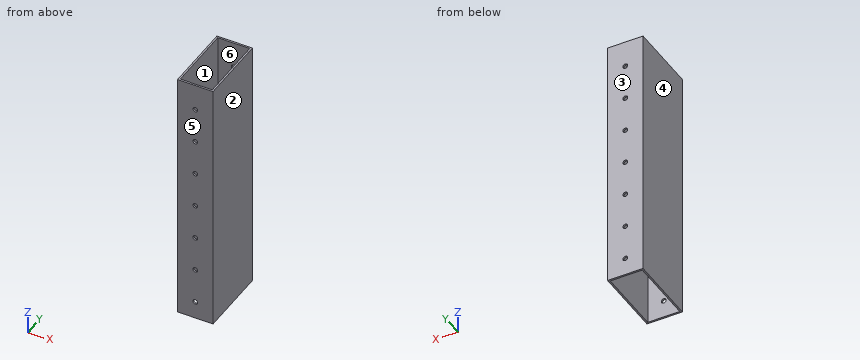
Autodesk Inventor part; units mm, degrees
ref_plane "YZ Plane" through (0, 0, 0) normal (1, 0, 0) x (0, 1, 0)
ref_plane "XZ Plane" through (0, 0, 0) normal (0, 1, 0) x (-1, 0, 0)
ref_plane "XY Plane" through (0, 0, 0) normal (0, 0, 1) x (1, 0, 0)
sketch "Sketch1" plane through (0, 0, 0) normal (0, 0, 1) x (1, 0, 0)
  line L0 (-12.1708, 16.0073) -> (13.2292, 16.0073)
  line L1 (13.2292, 16.0073) -> (13.2292, -34.7927)
  line L2 (13.2292, -34.7927) -> (-12.1708, -34.7927)
  line L3 (-12.1708, -34.7927) -> (-12.1708, 16.0073)
  line L4 (11.9592, 14.7373) -> (-10.9008, 14.7373)
  line L5 (-10.9008, 14.7373) -> (-10.9008, -33.5227)
  line L6 (-10.9008, -33.5227) -> (11.9592, -33.5227)
  line L7 (11.9592, -33.5227) -> (11.9592, 14.7373)
  point P0 (0, 0)
  dimension "d0" = 25.4
  dimension "d1" = 50.8
  dimension "d2" = 1.27
extrude "Extrusion1" add sketch "Sketch1" along normal blind 184.15
sketch "Sketch2" plane through (-12.1708, 16.0073, 0) normal (0, 1, 0) x (1, 0, 0)
  circle A0 centre (12.7, -12.7) radius 1.7272
  line L0 (25.4, 0) -> (0, 0)
  line L1 (0, 0) -> (0, -184.15)
  point P0 (12.1708, 0)
  dimension "d5" = 3.4544
  dimension "d6" = 12.7
  dimension "d7" = 12.7
extrude "Extrusion2" cut sketch "Sketch2" against normal through all
pattern_linear "Rectangular Pattern1" count 71 spacing 25.4 along (0, 0, 1) of "Extrusion2"
equation "\"d10\" = d14"
equation "\"d13\" = 711.2"
equation "\"d14\" = d13"
properties part number "VersaFrame_IndexSupp"
Geometry: final body of the model. Coordinates: model frame, mm. Face numbers are marked on the shaded views. A direction names the side the tool comes from. Coordinates: 2 decimals unless noted, no trailing zeros. Order: outer loops, then holes, each group sorted by start corner. A loop starts at its lowest first (then second) coordinate and runs counter-clockwise, first axis right, second up. Notation, with made-up numbers: M -29.5,29 L 7.5,29 A22 ccw 7.5,53 Z; hole C 76,46 d11. An arc over 180 degrees is marked long. Answer in a Markdown table with one row per item. Add a question column.
Q1. Line query: L1, parallel to X at y = -34.5, z = 165.1; L2, parallel to X at y = 15, z = 114; L3, parallel to Y at x = 9.25, z = 120. Output: solid intervals per line, ascending.
Q2. Contact query for a flat-ended pin moving along its axis: P1, Ø3, axis at x = 0.53, z = 12.7, coming from the +Y side. Output: stop coordinate, or through.
Q3. Mould query, pull axis Y, two halves, no side actions, for the marked faces 3, 4, 5 and 6. Classes: released by +Y, released by -Y, zero draft, split by the parting line, or undercut.
Q4. Section query C-C on x = 8.75. Return the cut outline in (y, z).
Q5. Section query B-B on y = 11.5. Return the cut outline in (x, z), and give its area (3 significant figures).
Q6. Section query A-A on z = 12.7. Return the cut outline in (x, y).
Q7. Section query D-D on z = 48.5. Return the cut outline in (x, y).
Q8. Reachability of the marked faces 1 and 2 from +Z, -Z, +X, -X, +Y, -Y: full face, straight path, thin tool, end or side. Return the list, or none.
Completed:
| question | item | result |
|---|---|---|
| 1 | L1 | x = -12.17 to -1.2, 2.26 to 13.23 |
| 1 | L2 | x = -12.17 to -1.17, 2.23 to 13.23 |
| 1 | L3 | y = -34.79 to -33.52, 14.74 to 16.01 |
| 2 | P1 | passes through |
| 3 | face 3 | released by +Y |
| 3 | face 4 | zero draft |
| 3 | face 5 | released by -Y |
| 3 | face 6 | undercut |
| 4 | outline | M -34.79,0 L -33.52,0 L -33.52,184.15 L -34.79,184.15 Z; M 14.74,0 L 16.01,0 L 16.01,184.15 L 14.74,184.15 Z |
| 5 | outline | M -12.17,0 L -10.9,0 L -10.9,184.15 L -12.17,184.15 Z; M 11.96,0 L 13.23,0 L 13.23,184.15 L 11.96,184.15 Z |
| 5 | area | 468 mm2 |
| 6 | outline | M -12.17,-34.79 L -1.2,-34.79 L -1.2,-33.52 L -10.9,-33.52 L -10.9,14.74 L -1.2,14.74 L -1.2,16.01 L -12.17,16.01 Z; M 2.26,-34.79 L 13.23,-34.79 L 13.23,16.01 L 2.26,16.01 L 2.26,14.74 L 11.96,14.74 L 11.96,-33.52 L 2.26,-33.52 Z |
| 7 | outline | M -12.17,-34.79 L 13.23,-34.79 L 13.23,16.01 L -12.17,16.01 Z; hole M -10.9,-33.52 L 11.96,-33.52 L 11.96,14.74 L -10.9,14.74 Z |
| 8 | face 1 | +Z, -Z |
| 8 | face 2 | +Z, -Z, +X, +Y, -Y |
